Part model, mm, in its own coordinate system. A direction names the side the tool comes from. Round coordinates to 2 decimals unless told otherwise and drop trailing zeros. Write each loop counter-clockwise with the first axis right and the second up, starting at its lowest first coordinate (ties: lowest second). Pieces come first, ordered by that corner, then holes. Notation, with made-up numbers: (-38, 56) -> (-11, 56) arc R24 cw to (-11, 69) -> close; hole circle Ø5 at (57, 66.25). An arc over 180 degrees is marked (long way). Use CSV: the item, a comma, the result in double quotes. Start each with the question number.
(1) Saw through at B-B (x = -0.75). Give the cut face in (y, z) (3 decimals), plus the area to 3 significant figures.
(2) Two-plate mould, pull along Z, no slides. Class faces 4 (the flat face through (8, 3, 19.05)), 5 (the flat face through (8, 3, -19.05)), 6 (the flat face through (10, 0, 0)), 7 (the flat face through (-2, 2, -9.525)): released by +Z, released by -Z, zero draft, split by the parting line, or undercut.
(3) Saw through at A-A (z = 12.7). Give the cut face in (x, y), plus the area to 3 significant figures.
(4) Saw through at C-C (x = 6). Give the cut face in (y, z).
(5) Saw through at D-D (z = -11). Count the separate pieces of the cut face and the enclosed holes in it, plus the area to 3 significant figures.
(6) Drop flat-ended pins along their axis: pin 1 (5 mm diameter, centred on x = 9, z = 5, fed in from +Y); pin 2 (6 mm diameter, centred on x = 14.224, z = 12.7, fed in from +Y). Give the stop position or say it passes through.
(7) Which spindle directions (+Z, -Z, +X, -X, +Y, -Y) get a long thin tool onto all of the face, cutting with end or side? Do faces 1 (the flat face through (-2, 2, 9.525)), 2 (the flat face through (12, 4.75, 0)), 3 (the conical face through (16.86, 2.23, 12.11)). Say none if no direction does.
(8) Probe line 1 (Z direction, x = 1.75, y = 7) (3 decimals); line 2 (Z direction, x = 16.25, y = 3.75); line 3 (Z direction, x = 12.5, y = 3.75). List the from-to ranges inside material, lowest first. Write a range as [from, to].
```python
from build123d import *

# Parameters (mm, degrees)
SKETCH1_R                                    = 2.38125
EXTRUDE1_DEPTH                               = 19.05
CSK_FOR_10_FLAT_HEAD_MACHINE_SCREW1_AT_COUNT = 2
CSK_FOR_10_FLAT_HEAD_MACHINE_SCREW1_AT_PITCH = 25.4
CUT_EXTRUDE1_DEPTH                           = 19.05


with BuildPart() as part:
    # Sketch1 → Extrude1 (new, symmetric)
    with BuildSketch(Plane.XY):
        with BuildLine():
            Line((4.348688447, 4.7498), (20.6375, 4.7498))
            Line((20.6375, 4.7498), (20.6375, 0))
            Line((20.6375, 0), (0, 0))
            ThreePointArc((0, 0), (-3.219925902, 1.417615701), (-4.348688447, 4.7498))
            ThreePointArc((-4.348688447, 4.7498), (0, 8.73125), (4.348688447, 4.7498))
        make_face()
        with Locations(Location((0, 4.365625, 0), (0, 0, 180))):
            Circle(SKETCH1_R, mode=Mode.SUBTRACT)
    extrude(amount=EXTRUDE1_DEPTH, both=True)

    # Sketch6 → CSK for #10 Flat Head Machine Screw1 (revolve, cut)
    with BuildSketch(Plane(origin=(14.224, 4.7498, 12.7), x_dir=(0, 0, 1), z_dir=(1, 0, 0))):
        Polygon((0, 0), (0, 4.7498), (2.5527, 4.7498), (2.5527, 2.688180894), (4.8895, 0), align=None)
    csk_for_10_flat_head_machine_screw1 = revolve(axis=Axis((14.224, 11.0998, 12.7), (0, -1, 0)), mode=Mode.SUBTRACT)

    # CSK for #10 Flat Head Machine Screw1 at: CSK for #10 Flat Head Machine Screw1 ×2
    with Locations(*[(0, 0, -i * CSK_FOR_10_FLAT_HEAD_MACHINE_SCREW1_AT_PITCH) for i in range(1, CSK_FOR_10_FLAT_HEAD_MACHINE_SCREW1_AT_COUNT)]):
        add(csk_for_10_flat_head_machine_screw1, mode=Mode.SUBTRACT)

    # Sketch8 → Cut-Extrude1 (cut)
    with BuildSketch(Plane(origin=(0, 0, -9.525), x_dir=(-1, 0, 0), z_dir=(0, 0, -1))):
        with BuildLine():
            ThreePointArc((-4.348688447, 4.7498), (-3.219925902, 1.417615701), (0, 0))
            ThreePointArc((0, 0), (3.219925902, 7.313634299), (-4.348688447, 4.7498))
        make_face()
    extrude(amount=-CUT_EXTRUDE1_DEPTH, mode=Mode.SUBTRACT)


solid = part.part
```
Answers:
1,outline,"(0.065, -19.05) -> (2.106, -19.05) -> (2.106, -9.525) -> (0.065, -9.525) -> close; (0.065, 9.525) -> (2.106, 9.525) -> (2.106, 19.05) -> (0.065, 19.05) -> close; (6.626, -19.05) -> (8.666, -19.05) -> (8.666, -9.525) -> (6.626, -9.525) -> close; (6.626, 9.525) -> (8.666, 9.525) -> (8.666, 19.05) -> (6.626, 19.05) -> close"
1,area,"77.7 mm²"
2,face 4,"released by +Z"
2,face 5,"released by -Z"
2,face 6,"zero draft"
2,face 7,"undercut"
3,outline,"(0, 0) -> (11.67, 0) -> (11.67, 2.06) -> (9.33, 4.75) -> (4.35, 4.75) arc R4.37 ccw (long way) to start; (16.78, 0) -> (20.64, 0) -> (20.64, 4.75) -> (19.11, 4.75) -> (16.78, 2.06) -> close; hole circle Ø4.76 at (0, 4.37)"
3,area,"92.9 mm²"
4,outline,"(0, -19.05) -> (4.75, -19.05) -> (4.75, 19.05) -> (0, 19.05) -> close"
5,separate pieces,"2"
5,enclosed holes,"1"
5,area,"97.9 mm²"
6,pin 1,"stops at y = 4.75"
6,pin 2,"stops at y = 2.58"
7,face 1,"-X, +Y"
7,face 2,"+Z, -Z, +X, +Y"
7,face 3,"+Y"
8,line 1,"z = [-19.05, -9.525], [9.525, 19.05]"
8,line 2,"z = [-19.05, -16.17], [-9.23, 9.23], [16.17, 19.05]"
8,line 3,"z = [-19.05, -16.33], [-9.07, 9.07], [16.33, 19.05]"
